```python
from build123d import *

# Parameters (mm, degrees)
SKETCH_1_W          = 120
SKETCH_1_H          = 60
SKETCH_1_W_2        = 4
SKETCH_1_H_2        = 11.25
EXTRUDE_1_DEPTH     = 4
SKETCH_2_W          = 7.5
SKETCH_2_H          = 2.8
SKETCH_2_W_2        = 2
SKETCH_2_H_2        = 5
CUT_EXTRUDE_1_DEPTH = 4
CUT_EXTRUDE_2_DEPTH = 71.795480082
FILLET_1_R          = 2.5


with BuildPart() as part:
    # Эскиз1 → Бобышка-Вытянуть1 (new body)
    with BuildSketch(Plane.XY):
        Rectangle(SKETCH_1_W, SKETCH_1_H)
        with Locations((-62, -11.875)):
            Rectangle(SKETCH_1_W_2, SKETCH_1_H_2)
        with Locations((-62, 11.875)):
            Rectangle(SKETCH_1_W_2, SKETCH_1_H_2)
        with Locations((62, 11.875)):
            Rectangle(SKETCH_1_W_2, SKETCH_1_H_2)
        with Locations((62, -11.875)):
            Rectangle(SKETCH_1_W_2, SKETCH_1_H_2)
    extrude(amount=EXTRUDE_1_DEPTH)

    # Эскиз2 → Вырез-Вытянуть1 (cut)
    with BuildSketch(Plane.XY.offset(4)):
        with Locations((-56.25, 23.75)):
            Rectangle(SKETCH_2_W, SKETCH_2_H)
        with Locations((-55, 23.75)):
            Rectangle(SKETCH_2_W_2, SKETCH_2_H_2)
        with Locations((55, 23.75)):
            Rectangle(SKETCH_2_W_2, SKETCH_2_H_2)
        with Locations((56.25, 23.75)):
            Rectangle(SKETCH_2_W, SKETCH_2_H)
        with Locations((56.25, -23.75)):
            Rectangle(SKETCH_2_W, SKETCH_2_H)
        with Locations((55, -23.75)):
            Rectangle(SKETCH_2_W_2, SKETCH_2_H_2)
        with Locations((-55, -23.75)):
            Rectangle(SKETCH_2_W_2, SKETCH_2_H_2)
        with Locations((-56.25, -23.75)):
            Rectangle(SKETCH_2_W, SKETCH_2_H)
    extrude(amount=-CUT_EXTRUDE_1_DEPTH, mode=Mode.SUBTRACT)

    # Эскиз3 → Вырез-Вытянуть2 (cut, through all)
    with BuildSketch(Plane.XY.offset(4)):
        Polygon((-47.5, 21.384101608), (-10.077822185, 0), (-47.5, -21.384101608), align=None)
        Polygon((-29.297177815, 22.5), (0, 5.758755534), (29.297177815, 22.5), align=None)
        Polygon((47.5, -21.384101608), (10.077822185, 0), (47.5, 21.384101608), align=None)
        Polygon((-29.297177815, -22.5), (0, -5.758755534), (29.297177815, -22.5), align=None)
    extrude(amount=-CUT_EXTRUDE_2_DEPTH, mode=Mode.SUBTRACT)

    # Скругление1
    fillet_1_edges = [part.edges().sort_by_distance(p)[0] for p in [
        (47.5, -21.384101608, 2),
        (10.077822185, 0, 2),
        (47.5, 21.384101608, 2),
        (0, 5.758755534, 2),
        (-29.297177815, 22.5, 2),
        (29.297177815, 22.5, 2),
        (-29.297177815, -22.5, 2),
        (0, -5.758755534, 2),
        (29.297177815, -22.5, 2),
        (-47.5, 21.384101608, 2),
        (-10.077822185, 0, 2),
        (-47.5, -21.384101608, 2),
    ]]
    fillet(fillet_1_edges, radius=FILLET_1_R)


solid = part.part
```
Check sheet for the modelled part. Datum: model origin and axes. Units: mm. A direction names the side the tool comes from. Give positions to 0.01 mm unless a question says otherwise; leave off trailing zeros. Order: outer loops, then holes, each group sorted by start corner. A loop starts at its lowest first (then second) coordinate and runs counter-clockwise, first axis right, second up. Notation, with made-up numbers: M 58.5,55 L 88.5,55 A12 cw 88.5,72 Z; hole C 87,71.5 d8. An arc over 180 degrees is marked long. Answer in a Markdown table with one row per item. Add a question column.
Q1. Sectioned sample at D-D, the plane x = -27. Record the boundary of the cut face in (y, z), and give its area (3 significant figures).
Q2. Release check for a two-part mould opening along X. For faces 1 (the flat face through (-1, 30, 2)), 2 (the flat face through (52.5, 24, 2)), 3 (the cylindrical face through (0.02, -6.14, 1.97)) record: released by +X, released by -X, zero draft, split by the parting line, or undercut.
Q3. Sectioned sample at C-C, the plane z = 2.3. Count the separate pieces of the cut face and the enclosed holes in it, and give its area (3 significant figures).
Q4. Thickness scan on L1, parallel to X at y = -5, z = 1.1; L2, parallel to Y at x = -1.5, z = 3.6; L3, parallel to Y at x = 57.5, z = 1.3. Record the ranges inside material, lowest first.
Q5. Sectioned sample at B-B, the plane y = -8.5. Record the boundary of the cut face in (x, z), and give its area (3 significant figures).
Q6. Access from +Z, -Z, +X, -X, +Y, -Y to the whole of each face (thin tool, end or side, straight path). Record for faces 4 (the flat face through (-62, 6.25, 2)), 5 (the flat face through (60, 20, 2)), 6 (the flat face through (-60, 20, 2)).
Q7. Sectioned sample at A-A, the plane x = 41. Record the boundary of the cut face in (y, z), and give its area (3 significant figures).
Q8. Gauge pin test, flat end, axial feed: pin 1 Ø1.2 at (y, z) = (21.5, 2.5) entering from -X. Record the tip position at first contact, or that the pin passes through.
Verdict:
| question | item | result |
|---|---|---|
| 1 | outline | M -30,0 L -9.67,0 L -9.67,4 L -30,4 Z; M 9.67,0 L 30,0 L 30,4 L 9.67,4 Z |
| 1 | area | 163 mm² |
| 2 | face 1 | zero draft |
| 2 | face 2 | released by +X |
| 2 | face 3 | undercut |
| 3 | separate pieces | 1 |
| 3 | enclosed holes | 4 |
| 3 | area | 4,780 mm² |
| 4 | L1 | -60 to -47.5, -18.83 to 18.83, 47.5 to 60 |
| 4 | L2 | -30 to -22.5, -6.62 to 6.62, 22.5 to 30 |
| 4 | L3 | -30 to -25.15, -22.35 to 22.35, 25.15 to 30 |
| 5 | outline | M -64,0 L -47.5,0 L -47.5,4 L -64,4 Z; M -24.95,0 L -4.8,0 L -4.8,4 L -24.95,4 Z; M 4.8,0 L 24.95,0 L 24.95,4 L 4.8,4 Z; M 47.5,0 L 64,0 L 64,4 L 47.5,4 Z |
| 5 | area | 293 mm² |
| 6 | face 4 | +Z, -Z, -X |
| 6 | face 5 | +Z, -Z, +X, +Y |
| 6 | face 6 | +Z, -Z, -X, +Y |
| 7 | outline | M -30,0 L -17.67,0 L -17.67,4 L -30,4 Z; M 17.67,0 L 30,0 L 30,4 L 17.67,4 Z |
| 7 | area | 98.6 mm² |
| 8 | pin 1 | x = -60 |
